Work out the finished part from the listing and answer in its coordinate system (mm). Coordinates: 2 decimals unless noted, no trailing zeros. Loops run counter-clockwise (first coordinate to the right, second up) from the corner with the lowest first, then second, coordinate; pieces in that order, holes last. Notation, with made-up numbers: M -21.75,67 L 30.25,67 A24 ccw 30.25,87 Z; hole C 75,23.25 d7. An arc over 180 degrees is marked long. Write each question's results on one line, items separated by ' | '.
```python
from build123d import *

# Parameters (mm, degrees)
SKETCH1_R           = 3.6703
BOSS_EXTRUDE1_DEPTH = 2.032


with BuildPart() as part:
    # Sketch1 → Boss-Extrude1 (new body)
    with BuildSketch(Plane(origin=(0, 0, 0), x_dir=(1, 0, 0), z_dir=(0, 1, 0))):
        Polygon((-2.764295354, 4.7879), (-5.528590708, 0), (-2.764295354, -4.7879), (2.764295354, -4.7879), (5.528590708, 0), (2.764295354, 4.7879), align=None)
        Circle(SKETCH1_R, mode=Mode.SUBTRACT)
    extrude(amount=BOSS_EXTRUDE1_DEPTH)

    # Sketch2 → Cut-Revolve1 (revolve, cut)
    with BuildSketch(Plane.XY):
        with BuildLine():
            Line((4.766590708, 2.032), (5.528590708, 2.032))
            Line((5.528590708, 2.032), (5.528590708, 1.27))
            ThreePointArc((5.528590708, 1.27), (5.305406075, 1.808815367), (4.766590708, 2.032))
        make_face()
        with BuildLine():
            Line((4.766590708, 0), (5.528590708, 0))
            Line((5.528590708, 0), (5.528590708, 0.762))
            ThreePointArc((5.528590708, 0.762), (5.305406075, 0.223184633), (4.766590708, 0))
        make_face()
    revolve(axis=Axis((0, 0, 0), (0, 1, 0)), mode=Mode.SUBTRACT)


solid = part.part
```
1) Given pin 1 Ø1 at (y, z) = (1, -2.5) entering from -X, flat-ended and moving along its own axis, determine where the tip first touches the part or whether it passes through.
Check result:
pin 1: x = -4.37
2) Find section C-C, the plane y = 1.7. Give the vertices of the cut face in (x, z), and give its area (3 significant figures).
Check result:
outline: M -5.39,-0.24 L -2.9,-4.55 A5.4 ccw -2.49,-4.79 L 2.49,-4.79 A5.4 ccw 2.9,-4.55 L 5.39,-0.24 A5.4 ccw 5.39,0.24 L 2.9,4.55 A5.4 ccw 2.49,4.79 L -2.49,4.79 A5.4 ccw -2.9,4.55 L -5.39,0.24 A5.4 ccw Z; hole C 0,0 d7.34 | area: 36.9 mm^2
3) For a pull along Z with two mould halves and no side action, classify faces 1 (the face through (-4.166, 1.002, 2.36)), 2 (the face through (1, 0, 4)), 3 (the face through (-3.667, 1.002, -0.161)), 4 (the face through (0, 1, -4.788)) as released by +Z, released by -Z, zero draft, split by the parting line, or undercut.
Check result:
face 1: released by +Z | face 2: zero draft | face 3: undercut | face 4: released by -Z
4) Find section B-B, the plane y = 0.25. Give the vertices of the cut face in (x, z), and give its area (3 significant figures).
Check result:
outline: M -5.32,-0.36 L -2.97,-4.42 A5.33 ccw -2.34,-4.79 L 2.34,-4.79 A5.33 ccw 2.97,-4.42 L 5.32,-0.36 A5.33 ccw 5.32,0.36 L 2.97,4.42 A5.33 ccw 2.34,4.79 L -2.34,4.79 A5.33 ccw -2.97,4.42 L -5.32,0.36 A5.33 ccw Z; hole C 0,0 d7.34 | area: 36.7 mm^2
5) Straight lines are drawn through the part: probe 1 along Z at (x, y) = (0, 0.7); probe 2 along X at (y, z) = (1.3, -0.5); probe 3 along X at (y, z) = (0.6, 0). For each, find the intervals that lie inside material, in ascending order. Write a range as [from, to].
Check result:
probe 1: [-4.79, -3.67], [3.67, 4.79] | probe 2: [-5.24, -3.64], [3.64, 5.24] | probe 3: [-5.51, -3.67], [3.67, 5.51]
